Autodesk Inventor part; units mm, degrees
ref_plane "YZ Plane" through (0, 0, 0) normal (1, 0, 0) x (0, 1, 0)
ref_plane "XZ Plane" through (0, 0, 0) normal (0, 1, 0) x (-1, 0, 0)
ref_plane "XY Plane" through (0, 0, 0) normal (0, 0, 1) x (1, 0, 0)
sketch "Sketch1" plane through (0, 0, 0) normal (0, 1, 0) x (-1, 0, 0)
  line L0 (-8.95, 8.85) -> (-8.95, -8.85)
  line L1 (-8.95, -8.85) -> (8.95, -8.85)
  line L2 (8.95, -8.85) -> (8.95, 8.85)
  line L3 (8.95, 8.85) -> (-8.95, 8.85)
  line L4 (-8.95, 8.85) -> (8.95, -8.85) construction
  line L5 (-8.95, -8.85) -> (8.95, 8.85) construction
  circle A0 centre (8.95, 8.85) radius 1.775
  circle A1 centre (8.95, -8.85) radius 1.775
  circle A2 centre (-8.95, 8.85) radius 1.775
  circle A3 centre (-8.95, -8.85) radius 1.775
  circle A4 centre (8.95, 8.85) radius 2.54
  circle A5 centre (8.95, -8.85) radius 2.54
  circle A6 centre (-8.95, 8.85) radius 2.54
  circle A7 centre (-8.95, -8.85) radius 2.54
  line L6 (2.2577, 2.2325) -> (2.2451, 2.2451)
  circle A8 centre (15.1, -15.1) radius 1.65
  circle A9 centre (15.1, 15.1) radius 1.65
  circle A10 centre (-15.1, -15.1) radius 1.65
  circle A11 centre (-15.1, 15.1) radius 1.65
  line L7 (0, 0) -> (4.4901, 0)
  line L8 (0, 0) -> (0, 3.0635)
  line L9 (-15.1, 15.1) -> (15.1, -15.1) construction
  circle A12 centre (15.1, 15.1) radius 3.175
  circle A13 centre (15.1, -15.1) radius 3.175
  circle A14 centre (-15.1, 15.1) radius 3.175
  circle A15 centre (-15.1, -15.1) radius 3.175
  line L10 (18.0638, 13.9613) -> (12.7, 0)
  line L11 (12.7, 0) -> (18.0638, -13.9613)
  line L12 (13.9613, 18.0638) -> (0, 12.7)
  line L13 (0, 12.7) -> (-13.9613, 18.0638)
  line L14 (-18.0638, 13.9613) -> (-12.7, 0)
  line L15 (-12.7, 0) -> (-18.0638, -13.9613)
  line L16 (-13.9613, -18.0638) -> (0, -12.7)
  line L17 (0, -12.7) -> (13.9613, -18.0638)
  point P0 (0, -0.2784)
  point P1 (-0.5887, -0.5887)
  point P2 (-4.5282, -4.9254)
  point P3 (0, 0)
  dimension "d0" = 17.7
  dimension "d1" = 17.9
  dimension "d2" = 3.55
  dimension "d3" = 3.55
  dimension "d4" = 3.55
  dimension "d5" = 3.55
  dimension "d11" = 5.08
  dimension "d12" = 5.08
  dimension "d13" = 5.08
  dimension "d14" = 5.08
  dimension "d31" = 3.3
  dimension "d34" = 30.2
  dimension "d37" = 30.2
  dimension "d68" = 6.35
  dimension "d71" = 30.2
  dimension "d74" = 30.2
  dimension "d78" = 12.7
  dimension "d79" = 12.7
  dimension "d81" = 12.7
extrude "Extrusion2" add sketch "Sketch1" along normal blind 10 contours L3 A2 L0 | L0 A2 L3 | A3 L1 L0 | L0 L1 A3 | A0 L2 L3 | L3 L2 A0 | A1 L2 L1 | L1 L2 A1
extrude "Extrusion3" add sketch "Sketch1" along normal blind 6 contours A2 L3 A6 L0 | L0 A6 L3 A2 | A7 L1 A3 L0 | L0 A3 L1 A7 | A4 L2 A0 L3 | L3 A0 L2 A4 | A5 L2 A1 L1 | L1 A1 L2 A5
extrude "Extrusion6" add sketch "Sketch1" along normal blind 2.5 contours L3 A2 L0 | A2 L3 A6 L0 | A6 L3 A4 L2 A5 L1 A7 L0 | A7 L1 A3 L0 | L3 A0 L2 A4 | A3 L1 L0 | L3 L2 A0 | A5 L2 A1 L1 | A1 L2 L1 | A12 | A12 L10 L11 A13 L17 L16 A15 L15 L14 A14 L13 L12 | A14 | A13 | A15 picked at (-7.7815, 8.7183) picked at (-6.6862, 8.6616) picked at (-6.6862, -8.6616) picked at (6.7011, 8.5299) picked at (-8.5616, -7.7401) picked at (7.7815, 8.7183) picked at (6.8287, -8.0375) picked at (8.8183, -7.6815)
fillet "Fillet2" radius 10 4 edges at (0, 1.25, 12.7) (12.7, 1.25, 0) (0, 1.25, -12.7) (-12.7, 1.25, 0)
fillet "Fillet3" radius 2 4 edges at (-6.41, 2.5, 8.85) (11.49, 2.5, 8.85) (11.49, 2.5, -8.85) (-6.41, 2.5, -8.85)
equation "\"d3\" = d2"
equation "\"d4\" = d2"
equation "\"d5\" = d2"
equation "\"d12\" = d11"
equation "\"d13\" = d11"
equation "\"d14\" = d11"
properties part number "Gryo Mount"
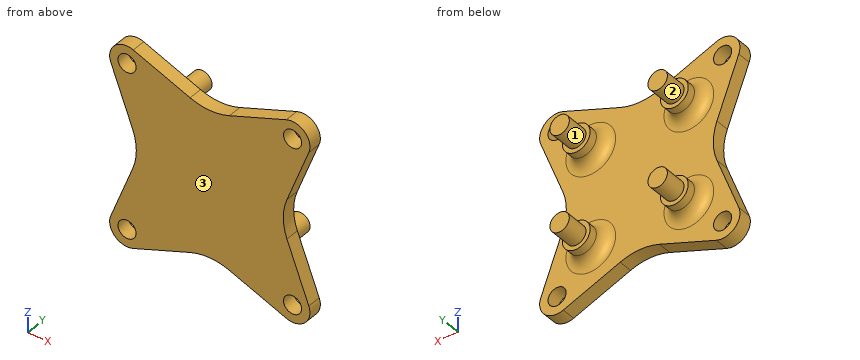
Verification items for the finished model (mm, model axes). Face numbers are marked on the shaded views. Give positions to 0.01 mm unless a question says otherwise; leave off trailing zeros. Write each loop counter-clockwise with the first axis right and the second up, starting at its lowest first coordinate (ties: lowest second). Pieces come first, ordered by that corner, then holes. Notation, with made-up numbers: (35.5, -31.75) - (63.5, -31.75) arc R9 ccw to (63.5, -16.75) - close; hole circle Ø2 at (-38, -9). An arc over 180 degrees is marked (long way). Answer as CSV lines item,"result". Start each with the question number.
1. Sectioned sample at C-C (y = 7.5). Record the boundary of the cut face in (x, z) (3 decimals), then the cut area to 3 significant figures.
2. Draft check along X on the marked faces 1, 2 and 3. Enter one of: pulls with the +X half, pulls with the -X half, needs draft (parallel to the pull), parting line crosses it, or undercut.
3. Depth check by flat-ended pin: pin 1 (1.5 mm diameter, centred on x = 11.5, y = 4, fed in from -Z); pin 2 (8 mm diameter, centred on x = 0, z = -8.5, fed in from +Y). Enter the tip coordinate at first touch or a pass-through.
4. Sectioned sample at A-A (z = 15.1). Record the boundary of the cut face in (x, y) (3 decimals).
5. Sectioned sample at B-B (y = 2). Record the boundary of the cut face in (x, z) (3 decimals), then the cut area to 3 significant figures.
6. Thickness scan on line 1 (Z direction, x = 9, y = 7.5); line 2 (Y direction, x = -16, z = 9); line 3 (X direction, y = 4.75, z = 9). Record the ranges inside material, lowest first.
7. Sectioned sample at D-D (x = 8.95). Record the boundary of the cut face in (y, z) (1 decimal), then the cut area to 3 significant figures.
Derived:
1,outline,"circle Ø3.55 at (-8.95, -8.85); circle Ø3.55 at (-8.95, 8.85); circle Ø3.55 at (8.95, -8.85); circle Ø3.55 at (8.95, 8.85)"
1,area,"39.6 mm²"
2,face 1,"undercut"
2,face 2,"undercut"
2,face 3,"needs draft"
3,pin 1,"z = -10.83"
3,pin 2,"y = 2.5"
4,outline,"(-18.275, 0) - (-16.75, 0) - (-16.75, 2.5) - (-18.275, 2.5) - close; (-13.45, 0) - (-6.247, 0) - (-6.247, 2.5) - (-13.45, 2.5) - close; (6.247, 0) - (13.45, 0) - (13.45, 2.5) - (6.247, 2.5) - close; (16.75, 0) - (18.275, 0) - (18.275, 2.5) - (16.75, 2.5) - close"
5,outline,"(-18.064, -13.961) arc R3.175 ccw to (-13.961, -18.064) - (-3.586, -14.078) arc R10 cw to (3.586, -14.078) - (13.961, -18.064) arc R3.175 ccw to (18.064, -13.961) - (14.078, -3.586) arc R10 cw to (14.078, 3.586) - (18.064, 13.961) arc R3.175 ccw to (13.961, 18.064) - (3.586, 14.078) arc R10 cw to (-3.586, 14.078) - (-13.961, 18.064) arc R3.175 ccw to (-18.064, 13.961) - (-14.078, 3.586) arc R10 cw to (-14.078, -3.586) - close; hole circle Ø3.3 at (-15.1, -15.1); hole circle Ø3.3 at (-15.1, 15.1); hole circle Ø3.3 at (15.1, -15.1); hole circle Ø3.3 at (15.1, 15.1)"
5,area,"976 mm²"
6,line 1,"-10.62 to -7.08, 7.08 to 10.62"
6,line 2,"0 to 2.5"
6,line 3,"-11.49 to -6.41, 6.41 to 11.49"
7,outline,"(0, -16.1) - (2.5, -16.1) - (2.5, -13.4) arc R2 cw to (4.5, -11.4) - (6, -11.4) - (6, -10.6) - (10, -10.6) - (10, -7.1) - (6, -7.1) - (6, -6.3) - (4.5, -6.3) arc R2 cw to (2.5, -4.3) - (2.5, 4.3) arc R2 cw to (4.5, 6.3) - (6, 6.3) - (6, 7.1) - (10, 7.1) - (10, 10.6) - (6, 10.6) - (6, 11.4) - (4.5, 11.4) arc R2 cw to (2.5, 13.4) - (2.5, 16.1) - (0, 16.1) - close"
7,area,"148 mm²"
